```python
from build123d import *

# Parameters (mm, degrees)
SKETCH1_R           = 250
SKETCH1_R_2         = 162.5
BOSS_EXTRUDE1_DEPTH = 9.5
SKETCH2_R           = 202.5
SKETCH2_R_2         = 180
CUT_EXTRUDE1_DEPTH  = 7
SKETCH3_R           = 5
CUT_EXTRUDE2_DEPTH  = 355.063553617


with BuildPart() as part:
    # Sketch1 → Boss-Extrude1 (new, symmetric)
    with BuildSketch(Plane(origin=(0, 0, 0), x_dir=(1, 0, 0), z_dir=(0, 1, 0))):
        with Locations(Location((0, 0, 0), (0, 0, 270))):
            Circle(SKETCH1_R)
        with Locations(Location((0, 0, 0), (0, 0, 270))):
            Circle(SKETCH1_R_2, mode=Mode.SUBTRACT)
    extrude(amount=BOSS_EXTRUDE1_DEPTH, both=True)

    # Sketch2 → Cut-Extrude1 (cut)
    with BuildSketch(Plane(origin=(0, 9.5, 0), x_dir=(1, 0, 0), z_dir=(0, 1, 0))):
        with Locations(Location((0, 0, 0), (0, 0, 270))):
            Circle(SKETCH2_R)
        with Locations(Location((0, 0, 0), (0, 0, 270))):
            Circle(SKETCH2_R_2, mode=Mode.SUBTRACT)
    extrude(amount=-CUT_EXTRUDE1_DEPTH, mode=Mode.SUBTRACT)

    # Sketch3 → Cut-Extrude2 (cut, through all)
    with BuildSketch(Plane(origin=(0, 9.5, 0), x_dir=(1, 0, 0), z_dir=(0, 1, 0))):
        with Locations(Location((111.25, 192.690652342, 0), (0, 0, 270))):
            Circle(SKETCH3_R)
        with Locations(Location((222.5, 0, 0), (0, 0, 270))):
            Circle(SKETCH3_R)
        with Locations(Location((-222.5, 0, 0), (0, 0, 90))):
            Circle(SKETCH3_R)
        with Locations(Location((-111.25, 192.690652342, 0), (0, 0, 90))):
            Circle(SKETCH3_R)
        with Locations(Location((111.25, -192.690652342, 0), (0, 0, 90))):
            Circle(SKETCH3_R)
        with Locations(Location((-111.25, -192.690652342, 0), (0, 0, 270))):
            Circle(SKETCH3_R)
    extrude(amount=-CUT_EXTRUDE2_DEPTH, mode=Mode.SUBTRACT)


solid = part.part
```
Part model, mm, in its own coordinate system. A direction names the side the tool comes from. Round coordinates to 2 decimals unless told otherwise and drop trailing zeros. Loops run counter-clockwise (first coordinate to the right, second up) from the corner with the lowest first, then second, coordinate; pieces in that order, holes last. Notation, with made-up numbers: (25, 76.25) -> (38, 76.25) arc R28 ccw to (38, 94.25) -> close; hole circle Ø3 at (29, 31). An arc over 180 degrees is marked (long way). Use CSV: the item, a comma, the result in double quotes. Start each with the question number.
1) Cut at A-A, the plane y = -6.5. Write the cut outline in (x, z), plus the area to 3 significant figures.
2) Drop flat-ended pins along their axis: P1, Ø5, axis at y = 6, z = 115.5, coming from the -X side; P2, Ø4, axis at y = -7, z = 31, coming from the +X side; P3, Ø1.5, axis at y = 6, z = -105.5, coming from the -X side. Give the stop position or say it passes through.
3) Wall check: L1, parallel to X at y = 3.25, z = 0; L2, parallel to X at y = -4, z = 0; L3, parallel to X at y = 4.25, z = 66.5. Give the ranges that are in metal, low to high. Write a range as [from, to].
4) Cut at D-D, the plane z = -215. Write the cut outline in (x, y).
5) Which spindle directions (+Z, -Z, +X, -X, +Y, -Y) get a long thin tool onto all of the face, cutting with end or side? Do faces 5 (the cylindrical face through (-197.685, 6.049, -43.898)), 6 (the flat face through (-163, -9.5, -4)). Say none if no direction does.
6) Cut at B-B, the plane x = 0. Write the cut outline in (y, z), plus the area to 3 significant figures.
7) Cut at C-C, the plane z = -38. Write the cut outline in (x, y), plus the area to 3 significant figures.
8) Pull direction Z, two halves, no side cores. Call faces 1 (the cylindrical face through (137.02, -0.13, 87.36)), 2 (the flat face through (1, 9.5, 203)), 3 (the flat face through (-119, 2.5, -136)), 4 (the cylindrical face through (10.99, 0.13, -249.76)): +Z half, -Z half, draft (parallel to the pull), parting line (faces both ways), or undercut.
Determined:
1,outline,"circle Ø500 at (0, 0); hole circle Ø10 at (-222.5, 0); hole circle Ø325 at (0, 0); hole circle Ø10 at (-111.25, -192.69); hole circle Ø10 at (-111.25, 192.69); hole circle Ø10 at (111.25, -192.69); hole circle Ø10 at (111.25, 192.69); hole circle Ø10 at (222.5, 0)"
1,area,"113,000 mm2"
2,P1,"stops at x = -223"
2,P2,"stops at x = 248.31"
2,P3,"stops at x = -227"
3,L1,"x = [-250, -227.5], [-217.5, -202.5], [-180, -162.5], [162.5, 180], [202.5, 217.5], [227.5, 250]"
3,L2,"x = [-250, -227.5], [-217.5, -162.5], [162.5, 217.5], [227.5, 250]"
3,L3,"x = [-240.99, -191.27], [-167.27, -148.27], [148.27, 167.27], [191.27, 240.99]"
4,outline,"(-127.57, -9.5) -> (127.57, -9.5) -> (127.57, 9.5) -> (-127.57, 9.5) -> close"
5,face 5,"+Y"
5,face 6,"+Z, -Z, +X, -X, -Y"
6,outline,"(-9.5, -250) -> (9.5, -250) -> (9.5, -202.5) -> (2.5, -202.5) -> (2.5, -180) -> (9.5, -180) -> (9.5, -162.5) -> (-9.5, -162.5) -> close; (-9.5, 162.5) -> (9.5, 162.5) -> (9.5, 180) -> (2.5, 180) -> (2.5, 202.5) -> (9.5, 202.5) -> (9.5, 250) -> (-9.5, 250) -> close"
6,area,"3,010 mm2"
7,outline,"(-247.1, -9.5) -> (-157.99, -9.5) -> (-157.99, 9.5) -> (-175.94, 9.5) -> (-175.94, 2.5) -> (-198.9, 2.5) -> (-198.9, 9.5) -> (-247.1, 9.5) -> close; (157.99, -9.5) -> (247.1, -9.5) -> (247.1, 9.5) -> (198.9, 9.5) -> (198.9, 2.5) -> (175.94, 2.5) -> (175.94, 9.5) -> (157.99, 9.5) -> close"
7,area,"3,060 mm2"
8,face 1,"undercut"
8,face 2,"draft"
8,face 3,"undercut"
8,face 4,"parting line"
